Drawing for the job (mm, zero at the part's lowest x, y, z). Give positions to 0.01 mm unless a question says otherwise; leave off trailing zeros. Write each loop counter-clockwise with the first axis right and the second up, starting at its lowest first coordinate (ties: lowest second). Pieces come first, ordered by that corner, then holes. Notation, with made-up numbers: M -21.75,35 L 9.25,35 A22 ccw 9.25,69 Z; hole C -22,38 d1. An arc over 180 degrees is marked long. Use CSV: the item, a comma, the result in double quotes. Start each with the question number.
1. Drill centre lines: line 1 along Y through (x, z) = (34, 9.25); line 2 along Y through (x, z) = (6, 14); line 3 along Y through (x, z) = (34, 12.5). Where is each one in solid material? Low to high. Write a range as from..to.
2. Band-saw the part on C-C, the plane y = 7. List the corners of the cut face in (x, z).
3. Drop flat-ended pins along their axis: pin 1 Ø5.5 at (x, y) = (34.5, 29) entering from -Z; pin 2 Ø1.5 at (x, y) = (6.5, 6) entering from -Z; pin 3 Ø9 at (y, z) = (17.5, 15) entering from -X. Give the stop position or say it passes through.
4. Mould opens along Y. For the marked faces 1, 2, 3 and 4 say: pulls with the +Y half, pulls with the -Y half, needs draft (parallel to the pull), parting line crosses it, or undercut.
5. Band-saw the part on A-A, the plane z = 15. List the corners of the cut face in (x, y), then the cut area to 3 significant figures.
6. Band-saw the part on B-B, the plane y = 17.5. List the corners of the cut face in (x, z), then the cut area to 3 significant figures.
7. Band-saw the part on D-D, the plane x = 13. List the corners of the cut face in (y, z), then the cut area to 3 significant figures.
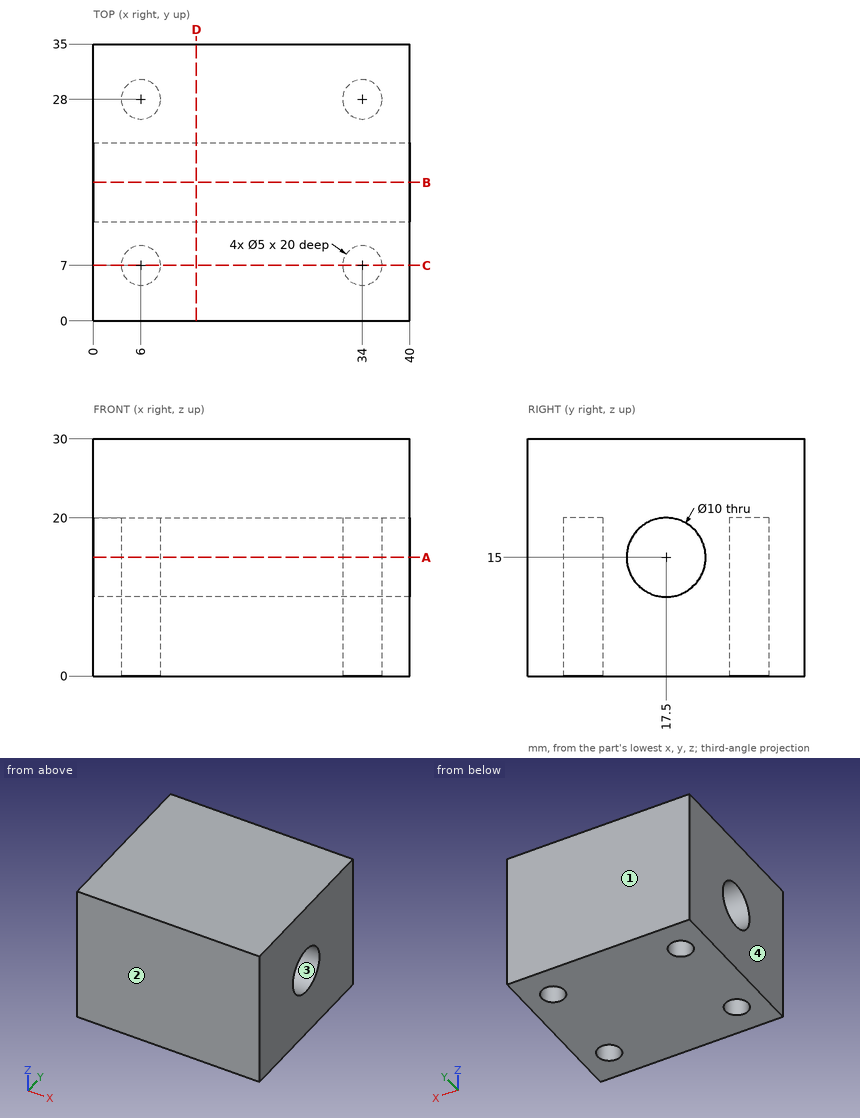
Output:
1,line 1,"y = 0..4.5, 9.5..25.5, 30.5..35"
1,line 2,"y = 0..4.5, 9.5..12.6, 22.4..25.5, 30.5..35"
1,line 3,"y = 0..4.5, 9.5..13.17, 21.83..25.5, 30.5..35"
2,outline,"M 0,0 L 3.5,0 L 3.5,20 L 8.5,20 L 8.5,0 L 31.5,0 L 31.5,20 L 36.5,20 L 36.5,0 L 40,0 L 40,30 L 0,30 Z"
3,pin 1,"stops at z = 0"
3,pin 2,"stops at z = 20"
3,pin 3,"passes through"
4,face 1,"pulls with the +Y half"
4,face 2,"pulls with the -Y half"
4,face 3,"undercut"
4,face 4,"needs draft"
5,outline,"M 0,0 L 40,0 L 40,12.5 L 0,12.5 Z; M 0,22.5 L 40,22.5 L 40,35 L 0,35 Z; hole C 6,7 d5; hole C 6,28 d5; hole C 34,7 d5; hole C 34,28 d5"
5,area,"921 mm²"
6,outline,"M 0,0 L 40,0 L 40,10 L 0,10 Z; M 0,20 L 40,20 L 40,30 L 0,30 Z"
6,area,"800 mm²"
7,outline,"M 0,0 L 35,0 L 35,30 L 0,30 Z; hole C 17.5,15 d10"
7,area,"971 mm²"
